from build123d import *

# Parameters (mm, degrees)
BOSS_EXTRUDE1_DEPTH = 1.143
SKETCH2_W           = 0.889
SKETCH2_H           = 8.243996394
BOSS_EXTRUDE2_DEPTH = 1.016
CHAMFER1_SIZE       = 1.27


with BuildPart() as part:
    # Sketch1 → Boss-Extrude1 (new body)
    with BuildSketch(Plane.XY):
        Polygon((37.147499812, 66.75804972), (39.128699766, 66.758049722), (39.128699766, 66.16665148), (42.151299766, 66.166651485), (42.151299766, 66.758049727), (44.132499719, 66.758049729), (44.13249971, 73.743049637), (42.151299756, 73.743049634), (42.151299755, 74.334447876), (39.128699755, 74.334447872), (39.128699756, 73.74304963), (37.147499802, 73.743049628), align=None)
    extrude(amount=BOSS_EXTRUDE1_DEPTH)

    # Sketch2 → Boss-Extrude2 (add)
    with BuildSketch(Plane(origin=(0, 0, 0), x_dir=(-1, 0, 0), z_dir=(0, 0, -1))):
        with Locations((-40.639999755, 70.212449679)):
            Rectangle(SKETCH2_W, SKETCH2_H)
    extrude(amount=BOSS_EXTRUDE2_DEPTH)

    # Chamfer1
    chamfer1_edges = [part.edges().sort_by_distance(p)[0] for p in [
        (37.147499802, 73.743049628, 0.5715),
        (44.13249971, 73.743049637, 0.5715),
        (44.132499719, 66.758049729, 0.5715),
        (37.147499812, 66.75804972, 0.5715),
    ]]
    chamfer(chamfer1_edges, length=CHAMFER1_SIZE)


solid = part.part
Part model, mm, in its own coordinate system. A direction names the side the tool comes from. Round coordinates to 2 decimals unless told otherwise and drop trailing zeros. Write each loop counter-clockwise with the first axis right and the second up, starting at its lowest first coordinate (ties: lowest second). Pieces come first, ordered by that corner, then holes. Notation, with made-up numbers: M -18,-17 L 17,-17 A19 ccw 17,-7 Z; hole C 27,18.5 d5. An arc over 180 degrees is marked long. Return JSON: item names as keys, results as strings. Group by question number.
(1) Saw through at B-B on z = 0.25. Write the cut outline in (x, y).
(2) Saw through at A-A on y = 70.75. Write the cut outline in (x, z).
(3) Pin check, flat tips, straight feed: pin 1 Ø1.5 at (x, y) = (42.5, 68) entering from -Z; pin 2 Ø3.5 at (x, y) = (39, 72) entering from -Z; pin 3 Ø0.5 at (y, z) = (70.5, -0.5) entering from -X; pin 4 Ø0.6 at (x, z) = (42.5, 0.5) entering from +Y. Stop position of each tip, or through.
(4) Drill centre lines: probe 1 along Y at (x, z) = (39.5, 0.9); probe 2 along Z at (x, y) = (41.75, 69); probe 3 along X at (y, z) = (72.5, -0.6). Where is each one in solid material? Low to high.
(5) Saw through at D-D on x = 39. Write the cut outline in (y, z).
(6) Saw through at C-C on y = 66.5. Write the cut outline in (x, z), then the cut area to 3 significant figures.
(7) Which spindle directions (+Z, -Z, +X, -X, +Y, -Y) get a long thin tool onto all of the face, cutting with end or side? Do faces 1 (the face through (41, 70, 1.143)), 2 (the face through (39, 70, 0)), 3 (the face through (43, 70, 0)), 4 (the face through (40.6, 66.167, 0.6)). Say none if no direction does.
Returned:
{
 "1": {"outline": "M 37.15,68.03 L 38.42,66.76 L 39.13,66.76 L 39.13,66.17 L 42.15,66.17 L 42.15,66.76 L 42.86,66.76 L 44.13,68.03 L 44.13,72.47 L 42.86,73.74 L 42.15,73.74 L 42.15,74.33 L 39.13,74.33 L 39.13,73.74 L 38.42,73.74 L 37.15,72.47 Z"},
 "2": {"outline": "M 37.15,0 L 40.2,0 L 40.2,-1.02 L 41.08,-1.02 L 41.08,0 L 44.13,0 L 44.13,1.14 L 37.15,1.14 Z"},
 "3": {"pin 1": "z = 0", "pin 2": "z = -1.02", "pin 3": "x = 40.2", "pin 4": "y = 73.74"},
 "4": {"probe 1": "66.17 to 74.33", "probe 2": "0 to 1.14", "probe 3": "40.2 to 41.08"},
 "5": {"outline": "M 66.76,0 L 73.74,0 L 73.74,1.14 L 66.76,1.14 Z"},
 "6": {"outline": "M 39.13,0 L 40.2,0 L 40.2,-1.02 L 41.08,-1.02 L 41.08,0 L 42.15,0 L 42.15,1.14 L 39.13,1.14 Z", "area": "4.36 mm²"},
 "7": {"face 1": "+Z, +X, -X, +Y, -Y", "face 2": "-Z, -X, +Y, -Y", "face 3": "-Z, +X, +Y, -Y", "face 4": "+Z, +X, -X, -Y"}
}
